Autodesk Fusion 360 part; units mm, degrees
sketch "Sketch1" plane through (0, 0, 0) normal (0, 1, 0) x (1, 0, 0)
  line L0 (0, 0) -> (80, 0)
  line L1 (0, 0) -> (0, -65)
  line L2 (0, -65) -> (80, 0)
  dimension "d1" = 80
  dimension "d2" = 65
sketch "Sketch2" plane through (0, 0, 0) normal (0, 0, 1) x (1, 0, 0)
sketch "Sketch3" plane through (0, 0, 0) normal (0, 0, 1) x (1, 0, 0)
sketch "Sketch4" plane through (0, 0, 0) normal (0, 0, 1) x (1, 0, 0)
  line L0 (0, -15) -> (65, -15)
  arc A0 (65, -15) -> (65, 15) centre (65, 0) ccw
  line L1 (65, 15) -> (0, 15)
  arc A1 (0, 15) -> (0, -15) centre (0, 0) ccw
  line L2 (0, 0) -> (65, 0) construction
  dimension "d10" = 65
  dimension "d11" = 30
extrude "Extrude2" add sketch "Sketch4" along normal blind 4
sketch "Sketch5" plane through (0, 0, 4) normal (0, 0, 1) x (-1, 0, 0)
  arc A0 (0, -15) -> (0, 15) centre (0, 0) ccw
  line L0 (0, 15) -> (-65, 15)
  arc A1 (-65, 15) -> (-65, -15) centre (-65, 0) ccw
  line L1 (-65, -15) -> (0, -15)
sketch "Sketch6" plane through (0, 0, 4) normal (0, 0, 1) x (-1, 0, 0)
sketch "Sketch7" plane through (0, 0, 4) normal (0, 0, 1) x (-1, 0, 0)
  line L0 (-80, -15) -> (-52, -15)
  line L1 (-52, -15) -> (-52, -7)
  line L2 (-52, -7) -> (-80, -7)
  line L3 (-80, -7) -> (-80, -15)
  dimension "d18" = 28
  dimension "d19" = 8
extrude "Extrude3" cut sketch "Sketch7" against normal blind 4
sketch "Sketch8" plane through (0, 0, 4) normal (0, 0, 1) x (-1, 0, 0)
  circle A0 centre (0, 0) radius 3
  dimension "d22" = 6
extrude "Extrude4" cut sketch "Sketch8" against normal blind 4
fillet "Fillet1" radius 1.5 8 edges at (26, 15, 4) (-15, 0, 4) (32.5, -15, 4) (77.8452, -7.746, 4) (26, 15, 0) (-15, 0, 0) (32.5, -15, 0) (77.8452, -7.746, 0)
fillet "Fillet2" radius 1 2 edges at (2.797, 1.0848, 0) (2.797, -1.0848, 4)
Can you work these out from the model? Positions are in its coordinate system, mm. A direction names the side the tool comes from. Give positions to 0.01 mm unless a question says otherwise; leave off trailing zeros. Order: outer loops, then holes, each group sorted by start corner. A loop starts at its lowest first (then second) coordinate and runs counter-clockwise, first axis right, second up. Notation, with made-up numbers: M 79.5,60.5 L 124.5,60.5 A29 cw 124.5,97.5 Z; hole C -5.75,-17.5 d1. An arc over 180 degrees is marked long. Use one line per item in the form item = value. Start each with the question number.
Item 1: If I drill on line 1 along X through (y, z) = (0, 1.65); line 2 along Y through (x, z) = (0, 1.4); line 3 along Y through (x, z) = (2.5, 3.5), over which ranges is the centre line in solid material (lowest first)?
Item 2: We'd pull the mould along Y, two halves only. Please class faces 3 (the cylindrical face through (25.64, 14.55, 3.57)), 4 (the flat face through (32, 0, 0)), 5 (the cylindrical face through (3, 0, 2)): +Y half, -Y half, draft (parallel to the pull), parting line (faces both ways), or undercut.
Item 3: For faces 1 (the flat face through (65, 7, 2)), 2 (the cylindrical face through (25.64, 14.57, 0.45)), which set-ups out of +Z, -Z, +X, -X, +Y, -Y let a thin tool reach every point of the face, with its end or its side?
Item 4: If we section it at A-A (x = 29.5): Write out the boundary of the cut face in (y, z).
Item 5: If we section it at B-B (x = 54.5): Write out the boundary of the cut face in (y, z).
Item 6: Will these pins go through, and if not, where does the flat tip stop? pin 1 Ø1.5 at (y, z) = (-5, 1) entering from -X; pin 2 Ø1 at (y, z) = (3, 3) entering from -X; pin 3 Ø1.5 at (x, y) = (54, 8.5) entering from +Z; pin 4 Ø1.5 at (x, y) = (-5, 7.5) entering from -Z.
Outcome:
q1.line_1 = -15 to -3, 3 to 80
q1.line_2 = -15 to -3, 3 to 15
q1.line_3 = -14.62 to -1.89, 1.89 to 14.62
q2.face_3 = +Y half
q2.face_4 = draft
q2.face_5 = undercut
q3.face_1 = +Z, -Z, +X, +Y
q3.face_2 = -Z, +X, -X, +Y
q4.outline = M -15,1.5 A1.5 ccw -13.5,0 L 13.5,0 A1.5 ccw 15,1.5 L 15,2.5 A1.5 ccw 13.5,4 L -13.5,4 A1.5 ccw -15,2.5 Z
q5.outline = M -15,1.5 A1.5 ccw -13.5,0 L 7,0 L 7,4 L -13.5,4 A1.5 ccw -15,2.5 Z
q6.pin_1 = -14.35
q6.pin_2 = -14.76
q6.pin_3 = through
q6.pin_4 = 0
